Can you work these out from the model? Positions are in its coordinate system, mm. Face numbers are marked on the shaded views. Coordinates: 2 decimals unless noted, no trailing zeros. Order: outer loops, then holes, each group sorted by start corner. A loop starts at its lowest first (then second) coordinate and runs counter-clockwise, first axis right, second up. Notation, with made-up numbers: M 1.25,-11 L 24.25,-11 A29 ccw 24.25,25 Z; hole C -5,79.5 d7. An arc over 180 degrees is marked long. Answer as a JSON object with one key per item and string values.
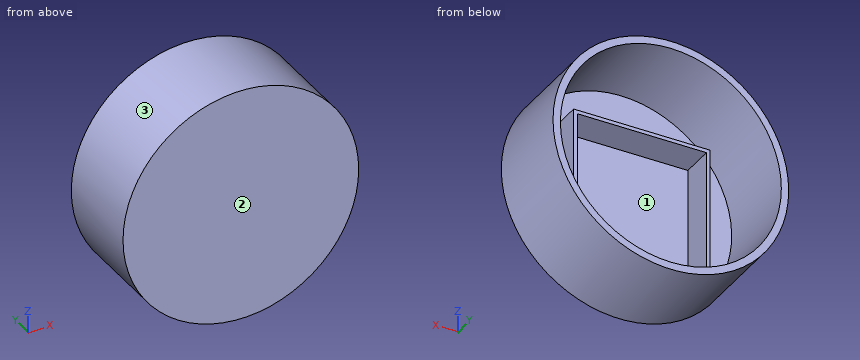
from build123d import *

# Parameters (mm, degrees)
SKETCH2_R           = 32
BOSS_EXTRUDE1_DEPTH = 25
SKETCH3_R           = 30
CUT_EXTRUDE1_DEPTH  = 24
BOSS_EXTRUDE2_DEPTH = 10
CUT_EXTRUDE2_DEPTH  = 9


with BuildPart() as part:
    # Sketch2 → Boss-Extrude1 (new body)
    with BuildSketch(Plane(origin=(0, 0, 0), x_dir=(1, 0, 0), z_dir=(0, 1, 0))):
        Circle(SKETCH2_R)
    extrude(amount=BOSS_EXTRUDE1_DEPTH)

    # Sketch3 → Cut-Extrude1 (cut)
    with BuildSketch(Plane(origin=(0, 25, 0), x_dir=(1, 0, 0), z_dir=(0, 1, 0))):
        Circle(SKETCH3_R)
    extrude(amount=-CUT_EXTRUDE1_DEPTH, mode=Mode.SUBTRACT)

    # Sketch4 → Boss-Extrude2 (add)
    with BuildSketch(Plane(origin=(0, 1, 0), x_dir=(1, 0, 0), z_dir=(0, 1, 0))):
        with BuildLine():
            Line((-18.541196676, -14.972239163), (18.541196676, -14.975032814))
            Line((18.541196676, -14.975032814), (18.541196676, 23.584402172))
            ThreePointArc((18.541196676, 23.584402172), (17.556036053, 24.32664379), (16.541196676, 25.027760837))
            Line((16.541196676, 25.027760837), (-16.541196676, 25.027760837))
            ThreePointArc((-16.541196676, 25.027760837), (-17.556036053, 24.32664379), (-18.541196676, 23.584402172))
            Line((-18.541196676, 23.584402172), (-18.541196676, -14.972239163))
        make_face()
    extrude(amount=BOSS_EXTRUDE2_DEPTH)

    # Sketch5 → Cut-Extrude2 (cut)
    with BuildSketch(Plane(origin=(0, 11, 0), x_dir=(1, 0, 0), z_dir=(0, 1, 0))):
        Polygon((-17.541196676, -13.973635989), (17.541196676, -13.973635989), (17.556036053, 24.32664379), (-17.556036053, 24.32664379), align=None)
    extrude(amount=-CUT_EXTRUDE2_DEPTH, mode=Mode.SUBTRACT)


solid = part.part
Item 1: If we mould it in two halves opening along X, with no side actions, what happens to the marked faces 1, 2 and 3? For each: pulls with the +X half, pulls with the -X half, needs draft (parallel to the pull), parting line crosses it, or undercut.
Answers follow:
{"face 1": "undercut", "face 2": "needs draft", "face 3": "parting line crosses it"}
Item 2: Please list where these lines run through material, in increasing order: line 1 (X direction, y = 7, z = 0); line 2 (Z direction, x = 0, y = 10.5); line 3 (X direction, y = 20, z = 0).
Answers follow:
{"line 1": "x = -32 to -30, -18.54 to -17.55, 17.55 to 18.54, 30 to 32", "line 2": "z = -32 to -30, -25.03 to -24.33, 13.97 to 14.97, 30 to 32", "line 3": "x = -32 to -30, 30 to 32"}
Item 3: I want a section at C-C, the plane z = -1. Write out the boundary of the cut face in (x, y), plus the area to 3 significant figures.
Answers follow:
{"outline": "M -31.98,0 L 31.98,0 L 31.98,25 L 29.98,25 L 29.98,1 L 18.54,1 L 18.54,11 L 17.55,11 L 17.55,2 L -17.55,2 L -17.55,11 L -18.54,11 L -18.54,1 L -29.98,1 L -29.98,25 L -31.98,25 Z", "area": "215 mm^2"}
Item 4: I want a section at B-B, the plane x = 23. Write out the boundary of the cut face in (y, z).
Answers follow:
{"outline": "M 0,-22.25 L 25,-22.25 L 25,-19.26 L 1,-19.26 L 1,19.26 L 25,19.26 L 25,22.25 L 0,22.25 Z"}
Item 5: I want a section at A-A, the plane y = 12.5. Write out the boundary of the cut face in (x, z).
Answers follow:
{"outline": "C 0,0 d64; hole C 0,0 d60"}
Item 6: I'm going to push flat-ended pins straight in: pin 1 (4 mm diameter, centred on y = 7, z = 9.5, fed in from +X); pin 2 (12 mm diameter, centred on x = 3, y = 5.5, fed in from +Z); pin 3 (0.6 mm diameter, centred on x = -6, z = -25, fed in from +Y). Where does each tip first touch, or does it pass through?
Answers follow:
{"pin 1": "stops at x = 31.11", "pin 2": "stops at z = 32", "pin 3": "stops at y = 11"}
Item 7: I want a section at D-D, the plane x = 7. Write out the boundary of the cut face in (y, z), plus the area to 3 significant figures.
Answers follow:
{"outline": "M 0,-31.22 L 25,-31.22 L 25,-29.17 L 1,-29.17 L 1,-25.03 L 11,-25.03 L 11,-24.33 L 2,-24.33 L 2,13.97 L 11,13.97 L 11,14.97 L 1,14.97 L 1,29.17 L 25,29.17 L 25,31.22 L 0,31.22 Z", "area": "216 mm^2"}
